Read the model definition and answer for the solid it produces. Units are mm, in the model's axes. Face numbers are marked on the shaded views. A direction names the side the tool comes from. Coordinates: 2 decimals unless noted, no trailing zeros. Loops run counter-clockwise (first coordinate to the right, second up) from the corner with the lowest first, then second, coordinate; pieces in that order, holes last.
from build123d import *

# Parameters (mm, degrees)
SKETCH_W                = 18.38
SKETCH_H                = 26
PAD_DEPTH               = 9.221
THICKNESS_T             = 1.6
SKETCH001_R             = 1.67005
PAD001_DEPTH            = 3.221
SKETCH001_MIRRORED_2_R  = 1.67005
PAD001_MIRRORED_2_DEPTH = 3.221
SKETCH002_R             = 3.3782
PAD002_DEPTH            = 1.6


with BuildPart() as part:
    # Sketch → Pad (new body)
    with BuildSketch(Plane.XY):
        Rectangle(SKETCH_W, SKETCH_H)
    extrude(amount=PAD_DEPTH)

    # Thickness
    thickness_openings = [part.faces().sort_by_distance(p)[0] for p in [
        (0, 0, 9.221),
    ]]
    offset(amount=THICKNESS_T, openings=thickness_openings)

    # Sketch001 → Pad001 (join)
    with BuildSketch(Plane.XY):
        with BuildLine():
            ThreePointArc((-6.35, 5.984875), (-3.397741, 7.207741), (-2.174875, 10.16))
            Line((-2.174875, 13), (-2.174875, 10.16))
            Line((-9.19, 13), (-2.174875, 13))
            Line((-9.19, 5.984875), (-9.19, 13))
            Line((-6.35, 5.984875), (-9.19, 5.984875))
        make_face()
        with Locations((-6.35, 10.16)):
            Circle(SKETCH001_R, mode=Mode.SUBTRACT)
    pad001 = extrude(amount=PAD001_DEPTH)

    # Sketch001 Mirrored 2 → Pad001 Mirrored 2 (add)
    with BuildSketch(Plane(origin=(0, 0, 0), x_dir=(-1, 0, 0), z_dir=(0, 0, -1))):
        with BuildLine():
            ThreePointArc((-6.35, 5.984875), (-3.397741, 7.207741), (-2.174875, 10.16))
            Line((-2.174875, 13), (-2.174875, 10.16))
            Line((-9.19, 13), (-2.174875, 13))
            Line((-9.19, 5.984875), (-9.19, 13))
            Line((-6.35, 5.984875), (-9.19, 5.984875))
        make_face()
        with Locations((-6.35, 10.16)):
            Circle(SKETCH001_MIRRORED_2_R, mode=Mode.SUBTRACT)
    pad001_mirrored_2 = extrude(amount=-PAD001_MIRRORED_2_DEPTH)

    # Mirrored001: Pad001, Pad001 Mirrored 2 across XZ
    add(pad001.mirror(Plane.XZ))
    add(pad001_mirrored_2.mirror(Plane.XZ))

    # Sketch002 → Pad002 (join)
    with BuildSketch(Plane.XY):
        with BuildLine():
            Line((-10.79, 32.8375), (-10.79, -32.8375))
            ThreePointArc((-10.79, -32.8375), (-10.204214, -34.251714), (-8.79, -34.8375))
            Line((-8.79, -34.8375), (8.79, -34.8375))
            ThreePointArc((8.79, -34.8375), (10.204214, -34.251714), (10.79, -32.8375))
            Line((10.79, -32.8375), (10.79, 32.8375))
            ThreePointArc((10.79, 32.8375), (10.204214, 34.251714), (8.79, 34.8375))
            Line((8.79, 34.8375), (-8.79, 34.8375))
            ThreePointArc((-8.79, 34.8375), (-10.204214, 34.251714), (-10.79, 32.8375))
        make_face()
        with Locations((0, 25.4)):
            Circle(SKETCH002_R, mode=Mode.SUBTRACT)
        with Locations((0, -25.4)):
            Circle(SKETCH002_R, mode=Mode.SUBTRACT)
    extrude(amount=-PAD002_DEPTH)


solid = part.part
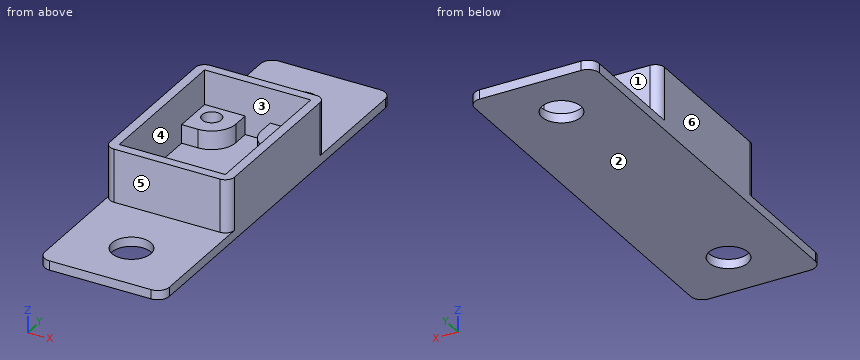
Q1. A cutting plane is placed at B-B (x = 0). Give the vertices of the cut face in (y, z).
Findings below:
outline: (-34.84, -1.6) - (-28.78, -1.6) - (-28.78, 0) - (-34.84, 0) - close; (-22.02, -1.6) - (22.02, -1.6) - (22.02, 0) - (14.6, 0) - (14.6, 9.22) - (13, 9.22) - (13, 0) - (-13, 0) - (-13, 9.22) - (-14.6, 9.22) - (-14.6, 0) - (-22.02, 0) - close; (28.78, -1.6) - (34.84, -1.6) - (34.84, 0) - (28.78, 0) - close
Q2. Flat-ended cylindrical pins translate along their axes: pin 1 Ø7.5 at (x, y) = (5, 8.5) entering from +Z; pin 2 Ø6.5 at (x, y) = (-1.5, 23) entering from +Z; pin 3 Ø3 at (x, z) = (1, 2.5) entering from +Y. Find the tip coordinate at first contact, or state that the pin passes through.
Findings below:
pin 1: stops at z = 3.22
pin 2: stops at z = 0
pin 3: stops at y = 14.6
Q3. A cutting plane is placed at D-D (y = 2.5). Give the vertices of the cut face in (x, z), then the cut area to 3 significant figures.
Findings below:
outline: (-10.79, -1.6) - (10.79, -1.6) - (10.79, 9.22) - (9.19, 9.22) - (9.19, 0) - (-9.19, 0) - (-9.19, 9.22) - (-10.79, 9.22) - close
area: 64.0 mm2
Q4. A cutting plane is placed at A-A (y = -25.4). Give the vertices of the cut face in (x, z).
Findings below:
outline: (-10.79, -1.6) - (-3.38, -1.6) - (-3.38, 0) - (-10.79, 0) - close; (3.38, -1.6) - (10.79, -1.6) - (10.79, 0) - (3.38, 0) - close
Q5. Determine the mould class of the marked faces 4, 5 and 6 for opening direction Y: +Y half, -Y half, draft (parallel to the pull), parting line (faces both ways), or undercut.
Findings below:
face 4: undercut
face 5: -Y half
face 6: draft
Q6. A cutting plane is placed at C-C (z = 2.5). Give the vertices of the cut face in (x, y), then the cut area to 3 significant figures.
Findings below:
outline: (-10.79, -13) arc R1.6 ccw to (-9.19, -14.6) - (9.19, -14.6) arc R1.6 ccw to (10.79, -13) - (10.79, 13) arc R1.6 ccw to (9.19, 14.6) - (-9.19, 14.6) arc R1.6 ccw to (-10.79, 13) - close; hole (-9.19, -5.98) - (-6.35, -5.98) arc R4.18 cw to (-2.17, -10.16) - (-2.17, -13) - (2.17, -13) - (2.17, -10.16) arc R4.18 cw to (6.35, -5.98) - (9.19, -5.98) - (9.19, 5.98) - (6.35, 5.98) arc R4.18 cw to (2.17, 10.16) - (2.17, 13) - (-2.17, 13) - (-2.17, 10.16) arc R4.18 cw to (-6.35, 5.98) - (-9.19, 5.98) - close; hole circle Ø3.34 at (-6.35, -10.16); hole circle Ø3.34 at (-6.35, 10.16); hole circle Ø3.34 at (6.35, -10.16); hole circle Ø3.34 at (6.35, 10.16)
area: 297 mm2
Q7. Which of the six approach directions +Z, -Z, +X, -X, +Y, -Y give full straight-line access (tool end or side, diameter ignored) to the marked faces 1, 2 and 3?
Findings below:
face 1: +Z, +X, -X, +Y
face 2: -Z, +X, -X, +Y, -Y
face 3: +Z
Q8. Straight lines are drawn through the part: probe 1 along Y at (x, z) = (-6.35, 1.25); probe 2 along Y at (x, z) = (0, -1.2); probe 3 along X at (y, z) = (-10.16, 1.4). For each, find the intervals that lie inside material, in ascending order.
Findings below:
probe 1: y = -14.6 to -11.83, -8.49 to -5.98, 5.98 to 8.49, 11.83 to 14.6
probe 2: y = -34.84 to -28.78, -22.02 to 22.02, 28.78 to 34.84
probe 3: x = -10.79 to -8.02, -4.68 to -2.17, 2.17 to 4.68, 8.02 to 10.79
